```python
from build123d import *

# Parameters (mm, degrees)
PAD_DEPTH    = 250
SKETCH001_W  = 2
SKETCH001_H  = 45
POCKET_DEPTH = 20


with BuildPart() as part:
    # Sketch → Pad (new body)
    with BuildSketch(Plane.XY):
        with BuildLine():
            Line((0, 0), (7.5, 0))
            Line((7.5, 0), (14.5, -9))
            Line((14.5, -9), (22, -9))
            Line((22, -9), (22, 1))
            Line((22, 1), (33, 1))
            ThreePointArc((33, 1), (34.680866, -3.511959), (38, -7))
            Line((38, -7), (38, -52))
            Line((38, -52), (25, -54))
            Line((25, -54), (25, -57))
            Line((25, -57), (12, -59))
            Line((12, -59), (12, -52))
            Line((12, -52), (0, -52))
            Line((0, -52), (0, 0))
        make_face()
    extrude(amount=PAD_DEPTH)

    # Sketch001 (on Face5 of Pad) → Pocket (cut)
    with BuildSketch(Plane(origin=(0, 1, 0), x_dir=(-1, 0, 0), z_dir=(0, 1, 0))):
        with Locations((-23, 102.5)):
            Rectangle(SKETCH001_W, SKETCH001_H)
    extrude(amount=-POCKET_DEPTH, mode=Mode.SUBTRACT)


solid = part.part
```
Model file for the job. Use its own axes, mm. A direction names the side the tool comes from. Coordinates: 2 decimals unless noted, no trailing zeros. Write each loop counter-clockwise with the first axis right and the second up, starting at its lowest first coordinate (ties: lowest second). Pieces come first, ordered by that corner, then holes. Notation, with made-up numbers: (-2.5, 69) - (21.5, 69) arc R35 cw to (21.5, 108) - close; hole circle Ø3 at (28, 59). An arc over 180 degrees is marked (long way). One line per item, written item: value. Start each with the question number.
1. Slice it at C-C (z = 122.5). Write the cut outline in (x, y), plus the area to 3 significant figures.
2. Flat gauge pins, fed straight in: pin 1 (1.6 mm diameter, centred on x = 22.5, z = 99.5, fed in from +Y); pin 2 (2 mm diameter, centred on x = 2.5, z = 182, fed in from +Y); pin 3 (3 mm diameter, centred on x = 33.5, z = 40, fed in from -Y). Where does each tip first touch, or does it go through?
3. Probe line 1 (Z direction, x = 22.5, y = -6); line 2 (X direction, y = -56, z = 12.5); line 3 (Y direction, x = 5.5, z = 237). List the from-to ranges inside material, lowest first. Write a range as from..to.
4. Tool access for faces 1 (the flat face through (4, 0, 123)), 2 (the flat face through (6, -52, 123)), 3 (the flat face through (18, -9, 123)), 4 (the flat face through (24, -9, 102)): list every direction of +Z, -Z, +X, -X, +Y, -Y with a clear straight run to the whole face (end or side of a thin tool).
5. Slice it at D-D (x = 17). Write the cut outline in (y, z).
6. Slice it at A-A (z = 23). Write the cut outline in (x, y), plus the area to 3 significant figures.
7. Slice it at B-B (x = 35.5). Write the cut outline in (y, z).
8. Mould opens along X. For faces 5 (the flat face through (31.591, -52.986, 123.25)), 6 (the flat face through (10.951, -4.437, 123.25)), 7 (the flat face through (12, -56, 123)) say: released by +X, released by -X, zero draft, split by the parting line, or undercut.
Answers below:
1. outline: (0, -52) - (12, -52) - (12, -59) - (25, -57) - (25, -54) - (38, -52) - (38, -7) arc R12 cw to (33, 1) - (24, 1) - (24, -19) - (22, -19) - (22, -9) - (14.5, -9) - (7.5, 0) - (0, 0) - close
1. area: 1,920 mm^2
2. pin 1: stops at y = -9
2. pin 2: stops at y = 0
2. pin 3: stops at y = -52.92
3. line 1: z = 0..80, 125..250
3. line 2: x = 12..25
3. line 3: y = -52..0
4. face 1: +Z, -Z, -X, +Y
4. face 2: +Z, -Z, -X, -Y
4. face 3: +Z, -Z, +Y
4. face 4: +Y
5. outline: (-58.23, 0) - (-9, 0) - (-9, 250) - (-58.23, 250) - close
6. outline: (0, -52) - (12, -52) - (12, -59) - (25, -57) - (25, -54) - (38, -52) - (38, -7) arc R12 cw to (33, 1) - (22, 1) - (22, -9) - (14.5, -9) - (7.5, 0) - (0, 0) - close
6. area: 1,960 mm^2
7. outline: (-52.38, 0) - (-4.67, 0) - (-4.67, 250) - (-52.38, 250) - close
8. face 5: released by +X
8. face 6: undercut
8. face 7: released by -X
